Geometry: final body of the model. Coordinates: model frame, mm. Face numbers are marked on the shaded views. A direction names the side the tool comes from. Give positions to 0.01 mm unless a question says otherwise; leave off trailing zeros. Write each loop counter-clockwise with the first axis right and the second up, starting at its lowest first coordinate (ties: lowest second). Pieces come first, ordered by that corner, then holes. Notation, with made-up numbers: (70.5, 9.25) -> (93.5, 9.25) arc R12 cw to (93.5, 25.25) -> close; hole circle Ø4 at (37.25, 75.25). An arc over 180 degrees is marked (long way). Answer as a JSON object with one key per item and string values.
from build123d import *

# Parameters (mm, degrees)
F1_R     = 2.185992
F3_W     = 3
F3_H     = 5.359665
F4_DEPTH = 2.8
F5_SIZE  = 1.65
F6_SIZE  = 1


with BuildPart() as f2:
    # F2: sweep along a path in F0
    with BuildLine(Plane.XY) as f2_path:
        ThreePointArc((0, 0), (5.5, 5.5), (0, 11))
        Line((0, 11), (-25, 11))
        ThreePointArc((-25, 11), (-30.5, 5.5), (-25, 0))
        Line((-25, 0), (0, 0))
    # F1 (on Right) → F2 (sweep)
    with BuildSketch(Plane.YZ):
        Circle(F1_R)
    sweep(path=f2_path.line)

    # F3 (on Top) → F4 (join, symmetric)
    with BuildSketch(Plane.XY):
        Polygon((-7.5, 2.841404), (-17.5, 2.841404), (-17.5, -3.153709), (-14.5, -3.153709), (-10.5, -3.153709), (-7.5, -3.153709), align=None)
        with Locations((-16, -5.833541)):
            Rectangle(F3_W, F3_H)
        with Locations((-9, -5.833541)):
            Rectangle(F3_W, F3_H)
    extrude(amount=F4_DEPTH, both=True)

    # F5
    f5_edges = [f2.edges().sort_by_distance(p)[0] for p in [
        (-12.5, 2.841404, 2.8),
        (-12.5, 2.841404, -2.8),
    ]]
    chamfer(f5_edges, length=F5_SIZE)

    # F6
    f6_edges = [f2.edges().sort_by_distance(p)[0] for p in [
        (-9, -8.513374, -2.8),
        (-7.5, -8.513374, 0),
        (-9, -8.513374, 2.8),
        (-16, -8.513374, -2.8),
        (-17.5, -8.513374, 0),
        (-16, -8.513374, 2.8),
    ]]
    chamfer(f6_edges, length=F6_SIZE)


solid = f2.part
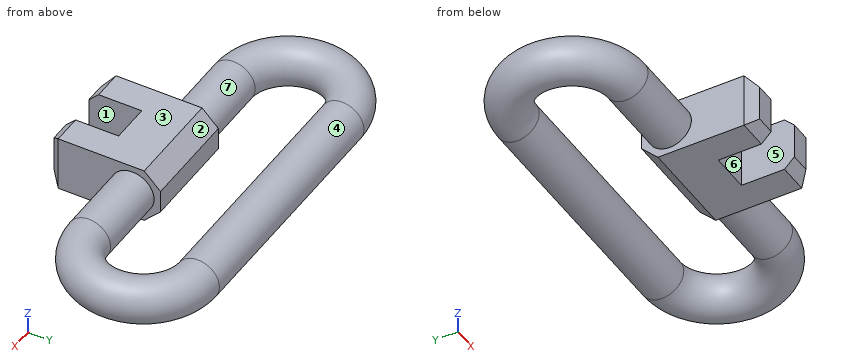
Q1. Cut plane C-C (y = -5.5). Return the cut outline in (x, z).
Values:
{"outline": "(-17.5, -2.8) -> (-14.5, -2.8) -> (-14.5, 2.8) -> (-17.5, 2.8) -> close; (-10.5, -2.8) -> (-7.5, -2.8) -> (-7.5, 2.8) -> (-10.5, 2.8) -> close"}
Q2. Material intervals for L1, parallel to X at y = -6.75, z = 1.45; L2, parallel to Y at x = -18, z = -0.15; L3, parallel to Z at x = -28.5, y = 10, sorted ascending. Write a range as from..to.
Values:
{"L1": "-17.5..-14.5, -10.5..-7.5", "L2": "-2.18..2.18, 8.82..13.18", "L3": "-2.18..2.18"}
Q3. Cut plane B-B (z = 0). Return the cut outline in (x, y), and give its area (3 significant figures).
Values:
{"outline": "(-25, -2.19) -> (-17.5, -2.19) -> (-17.5, -7.51) -> (-16.5, -8.51) -> (-14.5, -8.51) -> (-14.5, -3.15) -> (-10.5, -3.15) -> (-10.5, -8.51) -> (-8.5, -8.51) -> (-7.5, -7.51) -> (-7.5, -2.19) -> (0, -2.19) arc R7.69 ccw to (0, 13.19) -> (-25, 13.19) arc R7.69 ccw to start; hole (-25, 2.19) -> (-17.5, 2.19) -> (-17.5, 2.84) -> (-7.5, 2.84) -> (-7.5, 2.19) -> (0, 2.19) arc R3.31 ccw to (0, 8.81) -> (-25, 8.81) arc R3.31 ccw to start", "area": "417 mm²"}
Q4. Cut plane A-A (x = -13). Return the cut outline in (y, z).
Values:
{"outline": "(-3.15, -2.8) -> (1.19, -2.8) -> (2.84, -1.15) -> (2.84, 1.15) -> (1.19, 2.8) -> (-3.15, 2.8) -> close; circle Ø4.37 at (11, 0)"}
Q5. Set-up query: the marked faces 1, 2, 3 and 4. Return all of +Z, -Z, +X, -X, +Y, -Y with unobstructed straight access to the full face (end or side cutting, diameter ignored); none if empty.
Values:
{"face 1": "+Z, -Z, -Y", "face 2": "+Z", "face 3": "+Z, +X, -X, +Y, -Y", "face 4": "none"}
Q6. Cut plane D-D (x = -1). Return the cut outline in (y, z).
Values:
{"outline": "circle Ø4.37 at (0, 0); circle Ø4.37 at (11, 0)"}
Q7. First-contact query: P1, Ø1, axis at x = -13, z = -1, coming from the -Y side; P2, Ø1, axis at x = 0, y = 9, coming from the +Z side; P3, Ø6, axis at x = -4.5, y = 8, coming from the -Z side. Flat tips, straight axial feed; report the tip coordinate or a pass-through.
Values:
{"P1": "y = -3.15", "P2": "z = 1.59", "P3": "z = -2.19"}
Q8. Mould query, pull axis Y, two halves, no side actions, for the marked faces 5, 6 and 7. Classes: pulls with the +Y half, pulls with the -Y half, needs draft (parallel to the pull), parting line crosses it, or undercut.
Values:
{"face 5": "needs draft", "face 6": "pulls with the -Y half", "face 7": "undercut"}
